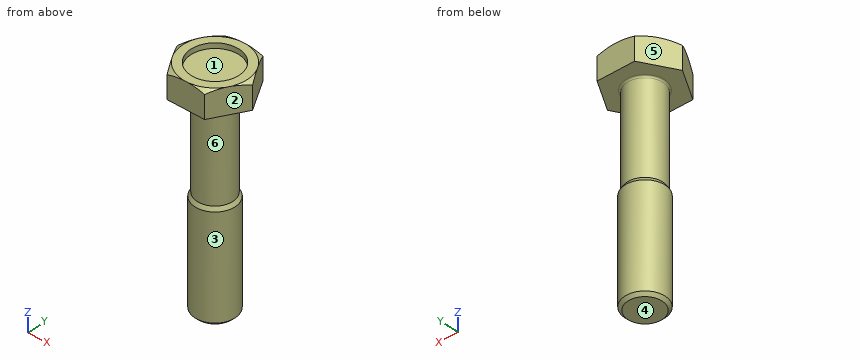
Autodesk Inventor part; units mm, degrees
ref_plane "MSC_PF1" through (0, 0, 0) normal (0, 1, 0) x (-1, 0, 0)
ref_plane "MSC_PT1" through (0, 0, 13.6501) normal (0, 0, -1) x (-1, 0, 0)
ref_plane "YZ Plane" through (0, 0, 0) normal (1, 0, 0) x (0, 1, 0)
sketch "Sketch2" plane through (0, 0, 0) normal (0, 1, 0) x (-1, 0, 0)
  line L0 (0, 13.6501) -> (0, -36.3499)
  line L1 (0, -36.3499) -> (4.25, -36.3499)
  line L2 (5, -35.5999) -> (5, -10.3499)
  line L3 (5, -10.3499) -> (4.45, -9.3972)
  line L4 (4.45, -9.3972) -> (4.45, 13.6501)
  line L5 (4.45, 13.6501) -> (0, 13.6501)
  line L6 (4.25, -36.3499) -> (5, -35.5999)
  line L7 (5, -36.3499) -> (5, -37.4105)
  line L8 (0, -47.6227) -> (0, 23.8623)
  dimension "Ds" = 8.9
  dimension "NND" = 10
  dimension "b" = 26
  dimension "d3" = 30
  dimension "d5" = 45
  dimension "PTC" = 1.5
  dimension "NLG" = 50
revolve "Revolution1" add sketch "Sketch2" angle 360 about axis through (0, 0, 13.6501) along (0, 0, -1)
sketch "Sketch3" plane through (0, 0, 13.6501) normal (0, 0, 1) x (1, 0, 0)
  circle A0 centre (0, 0) radius 4.45
  line L0 (0, 8) -> (4.6188, 8)
  line L1 (4.6188, 8) -> (9.2376, 0)
  line L2 (9.2376, 0) -> (0, 0)
  line L3 (0, 0) -> (0, 8)
  line L4 (0, 8) -> (-4.6188, 8)
  line L5 (-4.6188, 8) -> (-9.2376, 0)
  line L6 (0, -8) -> (4.6188, -8)
  line L7 (4.6188, -8) -> (9.2376, 0)
  line L8 (-4.6188, -8) -> (-9.2376, 0)
  line L9 (0, -8) -> (-4.6188, -8)
  dimension "d9" = 60
  dimension "ParS" = 16
  dimension "msp_d11" = 16
extrude "Extrusion1" add sketch "Sketch3" along normal blind 6.4
sketch "Sketch4" plane through (0, 0, 0) normal (0, 1, 0) x (-1, 0, 0)
  line L0 (-8, 20.0501) -> (-9.2376, 20.0501)
  line L1 (-9.2376, 20.0501) -> (-9.2376, 19.3356)
  line L2 (-9.2376, 19.3356) -> (-8, 20.0501)
  line L3 (0, 10.8015) -> (0, 30.7419)
  line L4 (0, 27.8933) -> (0, 27.1787)
  line L5 (-9.2376, 13.6501) -> (-9.2376, 20.0501)
  line L6 (-4.6188, 20.0501) -> (-9.2376, 20.0501)
  dimension "d14" = 30
  dimension "msp_d15" = 16
revolve "Revolution2" cut sketch "Sketch4" angle 360 about axis through (0, 0, 27.8933) along (0, 0, -1)
sketch "Sketch5" plane through (0, 0, 20.0501) normal (0, 0, 1) x (1, 0, 0)
  arc A0 (6.9282, 4) -> (0, 8) centre (0, 0) ccw
  circle A1 centre (0, 0) radius 6
  dimension "d27" = 12
extrude "Extrusion2" cut sketch "Sketch5" against normal blind 1.28
thread "Thread1"
ref_plane "MSC_PF1" through (0, 0, 0) normal (0, 1, 0) x (-1, 0, 0)
ref_plane "MSC_PT1" through (0, 0, 13.6501) normal (0, 0, -1) x (-1, 0, 0)
fillet "Fillet1" radius 0.4 1 edges at (4.45, 0, 13.6501)
equation "\"msp_d11\" = ParS"
equation "\"msp_d15\" = ParS"
equation "\"d27\" = 0.75 * ParS"
equation "\"d28\" = 0.2 * ParK"
equation "\"d30\" = r"
equation "\"msp_d17\" = b"
equation "\"r\" = 0.4"
properties part number "CSN EN 24015 - M10x50" material "Steel, Mild"
Work out the finished part from the listing and answer in its coordinate system (mm). Face numbers are marked on the shaded views. A direction names the side the tool comes from. Give positions to 0.01 mm unless a question says otherwise; leave off trailing zeros. Order: outer loops, then holes, each group sorted by start corner. A loop starts at its lowest first (then second) coordinate and runs counter-clockwise, first axis right, second up. Notation, with made-up numbers: (-38.75, 45) - (-1.75, 45) arc R17 cw to (-1.75, 73) - close; hole circle Ø2 at (46.25, 83). An arc over 180 degrees is marked (long way). One line per item, written item: value. Start each with the question number.
1. Consider line 1 (Y direction, x = 0, z = 19.7); line 2 (Z direction, x = -5, y = 6); line 3 (Z direction, x = 0.75, y = 2.75). Determine where each line is inside the solid, lowest interval first.
2. Section B-B, the plane z = -1 is taken. Write down the section's boundary in (x, y).
3. Which of the six approach directions +Z, -Z, +X, -X, +Y, -Y give full straight-line access (tool end or side, diameter ignored) to the marked faces 5 and 6?
4. Each of these flat-tipped pins is pushed along its axis until it touches: pin 1 Ø10 at (x, z) = (-5, 1) entering from -Y; pin 2 Ø9.5 at (x, y) = (0, -0.5) entering from +Z; pin 3 Ø8 at (x, z) = (2.5, -9.5) entering from +Y. Where does it stop, or does it pass through?
5. For a pull along X with two mould halves and no side action, classify the marked faces 1, 2, 3 and 4 as released by +X, released by -X, zero draft, split by the parting line, or undercut.
6. Section A-A, the plane z = -14.5 is taken. Write down the section's boundary in (x, y), then the cut area to 3 significant figures.
Filled sheet:
1. line 1: -8 to -6, 6 to 8
1. line 2: 13.65 to 20.05
1. line 3: -36.35 to 18.77
2. outline: circle Ø8.9 at (0, 0)
3. face 5: +Z, -Z, -X, +Y
3. face 6: none
4. pin 1: y = -4.45
4. pin 2: z = 18.77
4. pin 3: y = 5
5. face 1: undercut
5. face 2: released by +X
5. face 3: split by the parting line
5. face 4: zero draft
6. outline: circle Ø10 at (0, 0)
6. area: 78.5 mm²
